```python
from build123d import *

# Parameters (mm, degrees)
DISCO_START                         = 70
SK_DISCO_R                          = 65
DISCO_DEPTH                         = 6.35
CENTRADOR_ARANDELA_EJE_51110_START  = 67
SK_CENTRADOR_ARANDELA_EJE_51110_R   = 24.9
SK_CENTRADOR_ARANDELA_EJE_51110_R_2 = 23
CENTRADOR_ARANDELA_EJE_51110_DEPTH  = 3
PASANTES_M2_5_ROTOR_J1_START        = 70
SK_PASANTES_M2_5_ROTOR_J1_R         = 1.45
PASANTES_M2_5_ROTOR_J1_DEPTH        = 6.35
CAJAS_M2_5_START                    = 73.85
SK_CAJAS_M2_5_R                     = 2.75
CAJAS_M2_5_DEPTH                    = 2.5
PASO_CABLE_START                    = 70
SK_PASO_CABLE_R                     = 3
PASO_CABLE_DEPTH                    = 6.35
SK_PASANTES_M3_PAREDES_R            = 1.7
PASANTES_M3_PAREDES_DEPTH           = 93.398173683
SK_CAJAS_M3_PAREDES_R               = 3.25
CAJAS_M3_PAREDES_DEPTH              = 3.5


with BuildPart() as part:
    # Sk_Disco → Disco (new body)
    with BuildSketch(Plane.XY.offset(DISCO_START)):
        Circle(SK_DISCO_R)
    extrude(amount=DISCO_DEPTH)

    # Sk_Centrador_arandela_eje_51110 → Centrador_arandela_eje_51110 (add)
    with BuildSketch(Plane.XY.offset(CENTRADOR_ARANDELA_EJE_51110_START)):
        Circle(SK_CENTRADOR_ARANDELA_EJE_51110_R)
        Circle(SK_CENTRADOR_ARANDELA_EJE_51110_R_2, mode=Mode.SUBTRACT)
    extrude(amount=CENTRADOR_ARANDELA_EJE_51110_DEPTH)

    # Sk_Pasantes_M2-5_rotor_J1 → Pasantes_M2-5_rotor_J1 (cut)
    with BuildSketch(Plane.XY.offset(PASANTES_M2_5_ROTOR_J1_START)):
        with Locations((12.390194253, -1.653204878)):
            Circle(SK_PASANTES_M2_5_ROTOR_J1_R)
        with Locations((7.626814549, 9.903620542)):
            Circle(SK_PASANTES_M2_5_ROTOR_J1_R)
        with Locations((-4.763379704, 11.55682542)):
            Circle(SK_PASANTES_M2_5_ROTOR_J1_R)
        with Locations((-12.390194253, 1.653204878)):
            Circle(SK_PASANTES_M2_5_ROTOR_J1_R)
        with Locations((-7.626814549, -9.903620542)):
            Circle(SK_PASANTES_M2_5_ROTOR_J1_R)
        with Locations((4.763379704, -11.55682542)):
            Circle(SK_PASANTES_M2_5_ROTOR_J1_R)
    extrude(amount=PASANTES_M2_5_ROTOR_J1_DEPTH, mode=Mode.SUBTRACT)

    # Sk_Cajas_M2-5 → Cajas_M2-5 (cut)
    with BuildSketch(Plane.XY.offset(CAJAS_M2_5_START)):
        with Locations((12.390194253, -1.653204878)):
            Circle(SK_CAJAS_M2_5_R)
        with Locations((7.626814549, 9.903620542)):
            Circle(SK_CAJAS_M2_5_R)
        with Locations((-4.763379704, 11.55682542)):
            Circle(SK_CAJAS_M2_5_R)
        with Locations((-12.390194253, 1.653204878)):
            Circle(SK_CAJAS_M2_5_R)
        with Locations((-7.626814549, -9.903620542)):
            Circle(SK_CAJAS_M2_5_R)
        with Locations((4.763379704, -11.55682542)):
            Circle(SK_CAJAS_M2_5_R)
    extrude(amount=CAJAS_M2_5_DEPTH, mode=Mode.SUBTRACT)

    # Sk_Paso_cable → Paso_cable (cut)
    with BuildSketch(Plane.XY.offset(PASO_CABLE_START)):
        Circle(SK_PASO_CABLE_R)
    extrude(amount=PASO_CABLE_DEPTH, mode=Mode.SUBTRACT)

    # Sk_Pasantes_M3_paredes → Pasantes_M3_paredes (cut, through all)
    with BuildSketch(Plane.XY.offset(76.35)):
        with Locations((-42, -32.925)):
            Circle(SK_PASANTES_M3_PAREDES_R)
        with Locations((-20, -32.925)):
            Circle(SK_PASANTES_M3_PAREDES_R)
        with Locations((20, -32.925)):
            Circle(SK_PASANTES_M3_PAREDES_R)
        with Locations((42, -32.925)):
            Circle(SK_PASANTES_M3_PAREDES_R)
        with Locations((-42, 32.925)):
            Circle(SK_PASANTES_M3_PAREDES_R)
        with Locations((-20, 32.925)):
            Circle(SK_PASANTES_M3_PAREDES_R)
        with Locations((20, 32.925)):
            Circle(SK_PASANTES_M3_PAREDES_R)
        with Locations((42, 32.925)):
            Circle(SK_PASANTES_M3_PAREDES_R)
    extrude(amount=-PASANTES_M3_PAREDES_DEPTH, mode=Mode.SUBTRACT)

    # Sk_Cajas_M3_paredes → Cajas_M3_paredes (cut)
    with BuildSketch(Plane(origin=(0, 0, 70), x_dir=(-1, 0, 0), z_dir=(0, 0, -1))):
        with Locations((42, -32.925)):
            Circle(SK_CAJAS_M3_PAREDES_R)
        with Locations((20, -32.925)):
            Circle(SK_CAJAS_M3_PAREDES_R)
        with Locations((-20, -32.925)):
            Circle(SK_CAJAS_M3_PAREDES_R)
        with Locations((-42, -32.925)):
            Circle(SK_CAJAS_M3_PAREDES_R)
        with Locations((42, 32.925)):
            Circle(SK_CAJAS_M3_PAREDES_R)
        with Locations((20, 32.925)):
            Circle(SK_CAJAS_M3_PAREDES_R)
        with Locations((-20, 32.925)):
            Circle(SK_CAJAS_M3_PAREDES_R)
        with Locations((-42, 32.925)):
            Circle(SK_CAJAS_M3_PAREDES_R)
    extrude(amount=-CAJAS_M3_PAREDES_DEPTH, mode=Mode.SUBTRACT)


solid = part.part
```
Work out the finished part from the listing and answer in its coordinate system (mm). A direction names the side the tool comes from. Give positions to 0.01 mm unless a question says otherwise; leave off trailing zeros. Loops run counter-clockwise (first coordinate to the right, second up) from the corner with the lowest first, then second, coordinate; pieces in that order, holes last. Notation, with made-up numbers: (52.25, 6.25) -> (106.25, 6.25) arc R11 cw to (106.25, 22.25) -> close; hole circle Ø10 at (14.5, 25). An arc over 180 degrees is marked (long way). Write item = value, one per line. Start each with the question number.
(1) Find section D-D on x = 20. Give the vertices of the cut face in (y, z) (3 decimals), and give its area (3 significant figures).
(2) Which of the six approach directions +Z, -Z, +X, -X, +Y, -Y give full straight-line access (tool end or side, diameter ignored) to faces 1 (the cylindrical face through (-5.121, 14.283, 75.082)), 2 (the cylindrical face through (40.747, 34.074, 74.945)), 3 (the flat face through (-21.4, 31.5, 73.5))?
(3) The mould has two halves that part along Y. Classify faces 4 (the cylindrical face through (40.747, -31.776, 74.945)), 5 (the cylindrical face through (22.395, -30.728, 71.726)), 6 (the cylindrical face through (62, 19.52, 73.13)): +Y half, -Y half, draft (parallel to the pull), parting line (faces both ways), or undercut.
(4) Given pin 1 Ø2.5 at (x, y) = (8, 9) entering from +Z; pin 2 Ø1 at (y, z) = (48, 71) entering from +X; pin 3 Ø3 at (y, z) = (-32, 74) entering from -X, each flat-ended and moving along its own axis, determine where each tip first touches the part or whether it passes through.
(5) Find section B-B on z = 71.75. Give the number of separate pieces and of enclosed holes in the cut face, and give its area (3 significant figures).
(6) Find the intervals of material crossed by probe 1 along Y at (x, z) = (-20, 74.7) (3 decimals); probe 2 along X at (y, z) = (-30, 72.75); probe 3 along X at (y, z) = (-1, 70.25), in increasing order. Write a range as from..to.
(7) Find section A-A on x = 0. Give the vertices of the cut face in (y, z).
(8) Find section C-C on x = -42. Give the vertices of the cut face in (y, z) (3 decimals).
From the geometry:
q1.outline = (-61.847, 70) -> (-36.175, 70) -> (-36.175, 73.5) -> (-34.625, 73.5) -> (-34.625, 76.35) -> (-61.847, 76.35) -> close; (-31.225, 73.5) -> (-29.675, 73.5) -> (-29.675, 70) -> (-14.833, 70) -> (-14.833, 67) -> (-11.358, 67) -> (-11.358, 70) -> (11.358, 70) -> (11.358, 67) -> (14.833, 67) -> (14.833, 70) -> (29.675, 70) -> (29.675, 73.5) -> (31.225, 73.5) -> (31.225, 76.35) -> (-31.225, 76.35) -> close; (34.625, 73.5) -> (36.175, 73.5) -> (36.175, 70) -> (61.847, 70) -> (61.847, 76.35) -> (34.625, 76.35) -> close
q1.area = 741 mm^2
q2.face_1 = +Z
q2.face_2 = +Z, -Z
q2.face_3 = -Z
q3.face_4 = undercut
q3.face_5 = undercut
q3.face_6 = parting line
q4.pin_1 = 73.85
q4.pin_2 = 44.37
q4.pin_3 = -57.4
q5.separate_pieces = 1
q5.enclosed_holes = 15
q5.area = 12,900 mm^2
q6.probe_1 = -61.847..-34.625, -31.225..31.225, 34.625..61.847
q6.probe_2 = -57.66..-43.42, -40.58..-21.42, -18.58..18.58, 21.42..40.58, 43.42..57.66
q6.probe_3 = -64.99..-2.83, 2.83..11.1, 13.68..64.99
q7.outline = (-65, 70) -> (-24.9, 70) -> (-24.9, 67) -> (-23, 67) -> (-23, 70) -> (-3, 70) -> (-3, 76.35) -> (-65, 76.35) -> close; (3, 70) -> (23, 70) -> (23, 67) -> (24.9, 67) -> (24.9, 70) -> (65, 70) -> (65, 76.35) -> (3, 76.35) -> close
q8.outline = (-49.608, 70) -> (-36.175, 70) -> (-36.175, 73.5) -> (-34.625, 73.5) -> (-34.625, 76.35) -> (-49.608, 76.35) -> close; (-31.225, 73.5) -> (-29.675, 73.5) -> (-29.675, 70) -> (29.675, 70) -> (29.675, 73.5) -> (31.225, 73.5) -> (31.225, 76.35) -> (-31.225, 76.35) -> close; (34.625, 73.5) -> (36.175, 73.5) -> (36.175, 70) -> (49.608, 70) -> (49.608, 76.35) -> (34.625, 76.35) -> close
